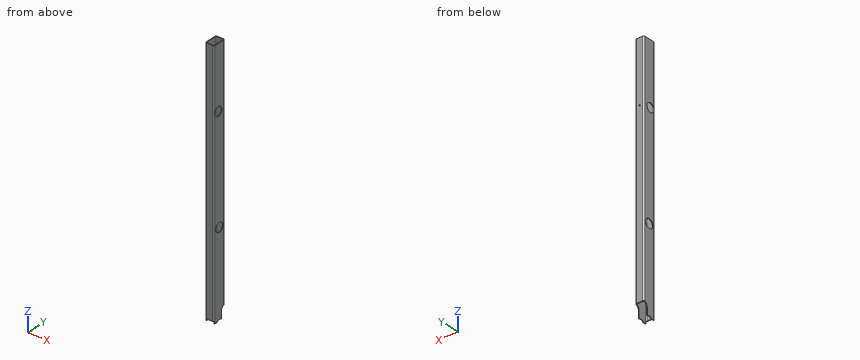
```python
from build123d import *

# Parameters (mm, degrees)
EXTRUDE_1_DEPTH     = 2865
SKETCH_4_R          = 50
CUT_EXTRUDE_3_DEPTH = 2871.666298963
SKETCH_3_R          = 50
SKETCH_3_R_2        = 51.5
SKETCH_3_W          = 25
SKETCH_3_H          = 10
CUT_EXTRUDE_2_DEPTH = 2871.666298963
FILLET_2_R          = 5
CUT_EXTRUDE_4_REACH = 2872.666
SKETCH_5_R          = 7.5


with BuildPart() as part:
    # 草图1 → 凸台-拉伸1 (new body)
    with BuildSketch(Plane.XY):
        with BuildLine():
            Line((16, 0), (84, 0))
            ThreePointArc((84, 0), (95.313708499, -4.686291501), (100, -16))
            Line((100, -16), (100, -134))
            ThreePointArc((100, -134), (95.313708499, -145.313708499), (84, -150))
            Line((84, -150), (16, -150))
            ThreePointArc((16, -150), (4.686291501, -145.313708499), (0, -134))
            Line((0, -134), (0, -16))
            ThreePointArc((0, -16), (4.686291501, -4.686291501), (16, 0))
        make_face()
        with BuildLine():
            Line((16, -8), (84, -8))
            ThreePointArc((84, -8), (89.656854249, -10.343145751), (92, -16))
            Line((92, -16), (92, -134))
            ThreePointArc((92, -134), (89.656854249, -139.656854249), (84, -142))
            Line((84, -142), (16, -142))
            ThreePointArc((16, -142), (10.343145751, -139.656854249), (8, -134))
            Line((8, -134), (8, -16))
            ThreePointArc((8, -16), (10.343145751, -10.343145751), (16, -8))
        make_face(mode=Mode.SUBTRACT)
    extrude(amount=-EXTRUDE_1_DEPTH)

    # 草图4 → 切除-拉伸3 (cut, through all)
    with BuildSketch(Plane(origin=(100, 0, 0), x_dir=(0, 0, -1), z_dir=(1, 0, 0))):
        with Locations((2900, -75)):
            Circle(SKETCH_4_R)
    extrude(amount=-CUT_EXTRUDE_3_DEPTH, mode=Mode.SUBTRACT)

    # 草图3 → 切除-拉伸2 (cut, through all)
    with BuildSketch(Plane(origin=(100, 0, 0), x_dir=(0, 0, -1), z_dir=(1, 0, 0))):
        with Locations(Location((700, -90.5, 0), (0, 0, 240.4586395))):
            Circle(SKETCH_3_R)
        with Locations(Location((1900, -75, 0), (0, 0, 90))):
            Circle(SKETCH_3_R_2)
        with BuildLine():
            Line((2775, -46), (2865, -46))
            Line((2865, -46), (2865, 0))
            Line((2865, 0), (2724.245689838, 0))
            ThreePointArc((2724.245689838, 0), (2740.750912421, -32.788887255), (2775, -46))
        make_face()
        with Locations((2852.5, -145)):
            Rectangle(SKETCH_3_W, SKETCH_3_H)
    extrude(amount=-CUT_EXTRUDE_2_DEPTH, mode=Mode.SUBTRACT)

    # 圆角2
    fillet_2_edges = [part.edges().sort_by_distance(p)[0] for p in [
        (94.061949798, -140, -2840),
    ]]
    fillet(fillet_2_edges, radius=FILLET_2_R)

    # 草图5 → 切除-拉伸4 (cut, up to next)
    with BuildSketch(Plane(origin=(0, 0, 0), x_dir=(1, 0, 0), z_dir=(0, 1, 0)), mode=Mode.PRIVATE) as cut_extrude_4_sk1:
        with Locations(Location((50, 700, 0), (0, 0, 270))):
            Circle(SKETCH_5_R)
    cut_extrude_4_tool1 = extrude(cut_extrude_4_sk1.sketch, amount=-CUT_EXTRUDE_4_REACH, mode=Mode.PRIVATE) & part.part
    add(cut_extrude_4_tool1.solids().sort_by_distance((50, 0, -700))[0], mode=Mode.SUBTRACT)


solid = part.part
```
Work out the finished part from the listing and answer in its coordinate system (mm). Round coordinates to 2 decimals unless told otherwise and drop trailing zeros. Write each loop counter-clockwise with the first axis right and the second up, starting at its lowest first coordinate (ties: lowest second). Pieces come first, ordered by that corner, then holes. Notation, with made-up numbers: (66, 6) - (106, 6) arc R6 cw to (106, 10) - close; hole circle Ø1 at (-28.75, 16.25). An arc over 180 degrees is marked (long way). Return JSON: item names as keys, results as strings. Group by question number.
Q1. Find the intervals of material crossed by L1, parallel to X at y = -124.5, z = -1120.5; L2, parallel to Y at x = 45, z = -398; L3, parallel to Z at x = 7, y = -90, in increasing order.
Q2. The part is cut by section A-A on z = -1900. Write down the section's boundary in (x, y).
Q3. Each of these flat-tipped pins is pushed along its axis until it touches: pin 1 Ø3 at (x, z) = (93, -2858) entering from -Y; pin 2 Ø6.5 at (x, z) = (4, -2819.5) entering from +Y; pin 3 Ø1.5 at (x, y) = (71.5, -148.5) entering from -Z. Where does it stop, or does it pass through?
Q4. The part is cut by section B-B on y = -75. Write down the section's boundary in (x, z).
Solved:
{
 "1": {"L1": "0 to 8, 92 to 100", "L2": "-150 to -142, -8 to 0", "L3": "-2852.3 to -1949.27, -1850.73 to -750, -650 to 0"},
 "2": {"outline": "(0, -134) arc R16 ccw to (16, -150) - (84, -150) arc R16 ccw to (100, -134) - (100, -126.5) - (92, -126.5) - (92, -134) arc R8 cw to (84, -142) - (16, -142) arc R8 cw to (8, -134) - (8, -126.5) - (0, -126.5) - close; (0, -23.5) - (8, -23.5) - (8, -16) arc R8 cw to (16, -8) - (84, -8) arc R8 cw to (92, -16) - (92, -23.5) - (100, -23.5) - (100, -16) arc R16 ccw to (84, 0) - (16, 0) arc R16 ccw to (0, -16) - close"},
 "3": {"pin 1": "y = -140", "pin 2": "y = -46", "pin 3": "z = -2840"},
 "4": {"outline": "(0, -2850) - (8, -2850) - (8, -1951.5) - (0, -1951.5) - close; (0, -1848.5) - (8, -1848.5) - (8, -747.54) - (0, -747.54) - close; (0, -652.46) - (8, -652.46) - (8, 0) - (0, 0) - close; (92, -2850) - (100, -2850) - (100, -1951.5) - (92, -1951.5) - close; (92, -1848.5) - (100, -1848.5) - (100, -747.54) - (92, -747.54) - close; (92, -652.46) - (100, -652.46) - (100, 0) - (92, 0) - close"}
}
